Can you work these out from the model? Positions are in its coordinate system, mm. Face numbers are marked on the shaded views. A direction names the side the tool comes from. Round coordinates to 2 decimals unless told otherwise and drop trailing zeros. Loops run counter-clockwise (first coordinate to the right, second up) from the corner with the lowest first, then second, coordinate; pieces in that order, holes last.
(1) Thinking about a two-plate mould opening in Y: for the marked faces 4, 5 and 6, which applies, released by +Y, released by -Y, zero draft, split by the parting line, or undercut?
(2) I want a section at C-C on x = 0.4. Write out the boundary of the cut face in (y, z).
(3) I want a section at B-B on z = 0.3. Write out the boundary of the cut face in (x, y).
(4) If I drill on line 1 along Y through (x, z) = (0.2, -0.25); line 2 along Y through (x, z) = (-0.6, 1.8); line 3 along X through (y, z) = (-11, 0.8), over which ranges is the centre line in solid material (lowest first)?
(5) I want a section at D-D on y = 2. Write out the boundary of the cut face in (x, z), plus the area to 3 significant figures.
(6) I want a section at A-A on y = 9. Write out the boundary of the cut face in (x, z).
(7) Will these pins go through, and if not, where does the flat tip stop? pin 1 Ø1.7 at (x, y) = (0.2, -11) entering from +Z; pin 2 Ø0.8 at (x, z) = (-1.5, 1) entering from +Y; pin 3 Ø0.6 at (x, y) = (0, 8) entering from +Z.
(8) Which directions (+Z, -Z, +X, -X, +Y, -Y) give clear straight access to the entire face, cutting with the end or side of a thin tool? Please do the marked faces 1, 2 and 3.
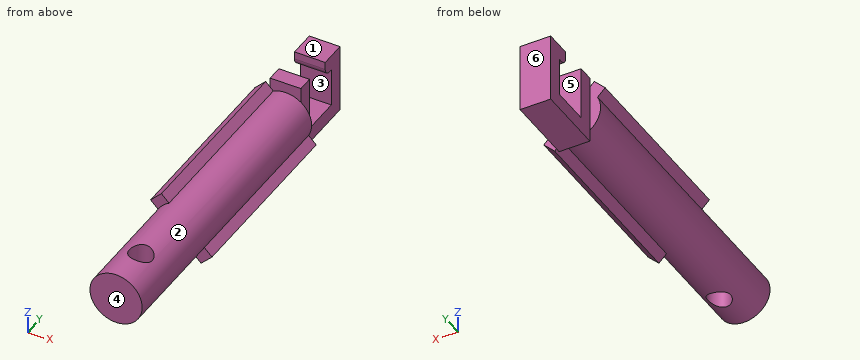
from build123d import *

# Parameters (mm, degrees)
SKETCH1_R             = 1.7
MAIN_SHAFT_DEPTH      = 6
GUIDES_DEPTH          = 12
SKETCH21_W            = 2
SKETCH21_H            = 4.5
HOOK_EXTRUDE_DEPTH    = 4.5
HOOK_CUT_DEPTH        = 3.997440667
HOOK_FILLET_R         = 0.5
SKETCH23_R            = 1.7
TOP_STOPPER_DEPTH     = 2
SKETCH24_R            = 1.7
BOTTOM_SHAFT_DEPTH    = 5.5
F_1_5MM_DOWEL_HOLE2_D = 1.5


with BuildPart() as part:
    # Sketch1 → main shaft (new body, symmetric)
    with BuildSketch(Plane(origin=(0, 0, 0), x_dir=(1, 0, 0), z_dir=(0, 1, 0))):
        Circle(SKETCH1_R)
    extrude(amount=MAIN_SHAFT_DEPTH, both=True)

    # Sketch2 → guides (add)
    with BuildSketch(Plane(origin=(0, 6, 0), x_dir=(1, 0, 0), z_dir=(0, 1, 0))):
        with BuildLine():
            Line((-0.795359139, -1.50246592), (-1.290333886, -1.997440667))
            Line((-1.290333886, -1.997440667), (-1.997440667, -1.290333886))
            Line((-1.997440667, -1.290333886), (-1.50246592, -0.795359139))
            ThreePointArc((-1.50246592, -0.795359139), (-1.202081528, -1.202081528), (-0.795359139, -1.50246592))
        make_face()
        with BuildLine():
            Line((1.290333886, 1.997440667), (0.795359139, 1.50246592))
            ThreePointArc((0.795359139, 1.50246592), (1.202081528, 1.202081528), (1.50246592, 0.795359139))
            Line((1.50246592, 0.795359139), (1.997440667, 1.290333886))
            Line((1.997440667, 1.290333886), (1.290333886, 1.997440667))
        make_face()
    extrude(amount=-GUIDES_DEPTH)

    # Sketch21 → hook extrude (add)
    with BuildSketch(Plane(origin=(0, 6, 0), x_dir=(1, 0, 0), z_dir=(0, 1, 0))):
        with Locations((0, -0.1)):
            Rectangle(SKETCH21_W, SKETCH21_H)
    extrude(amount=HOOK_EXTRUDE_DEPTH)

    # Sketch22 → hook cut (cut, through all)
    with BuildSketch(Plane(origin=(1, 0, 0), x_dir=(0, 0, -1), z_dir=(1, 0, 0))):
        Polygon((-2.35, 7), (1.15, 7), (1.15, 9.5), (-1.35, 9.5), (-1.35, 8.8), (-2.35, 8.8), align=None)
    extrude(amount=-HOOK_CUT_DEPTH, mode=Mode.SUBTRACT)

    # hook fillet
    hook_fillet_edges = [part.edges().sort_by_distance(p)[0] for p in [
        (0, 8.8, 1.35),
    ]]
    fillet(hook_fillet_edges, radius=HOOK_FILLET_R)

    # Sketch23 → top stopper (add)
    with BuildSketch(Plane.XZ.offset(6)):
        Circle(SKETCH23_R)
    extrude(amount=TOP_STOPPER_DEPTH)

    # Sketch24 → bottom shaft (add)
    with BuildSketch(Plane.XZ.offset(8)):
        Circle(SKETCH24_R)
    extrude(amount=BOTTOM_SHAFT_DEPTH)

    # Ø1.5mm Dowel Hole2 (through all)
    with Locations(Plane.XY.offset(2.35)):
        with Locations((0.2, -11)):
            Hole(F_1_5MM_DOWEL_HOLE2_D / 2)


solid = part.part
Filled sheet:
1. face 4: released by -Y
1. face 5: undercut
1. face 6: released by +Y
2. outline: (-13.5, -1.65) - (-11.72, -1.65) - (-11.72, 1.65) - (-13.5, 1.65) - close; (-10.28, -1.65) - (6, -1.65) - (6, -2.15) - (10.5, -2.15) - (10.5, 2.35) - (8.8, 2.35) - (8.8, 1.85) arc R0.5 ccw to (9.3, 1.35) - (9.5, 1.35) - (9.5, -1.15) - (7, -1.15) - (7, 2.35) - (6, 2.35) - (6, 1.65) - (-10.28, 1.65) - close
3. outline: (-1.67, -13.5) - (1.67, -13.5) - (1.67, 6) - (1, 6) - (1, 7) - (-1, 7) - (-1, 6) - (-1.67, 6) - close; (-1, 9.5) - (1, 9.5) - (1, 10.5) - (-1, 10.5) - close; hole circle Ø1.5 at (0.2, -11)
4. line 1: y = -13.5 to -11.75, -10.25 to 7, 9.5 to 10.5
4. line 2: y = 6 to 7, 8.8 to 10.5
4. line 3: x = -1.5 to -0.55, 0.95 to 1.5
5. outline: (-2, 1.29) - (-1.5, 0.8) arc R1.7 ccw to (0.8, -1.5) - (1.29, -2) - (2, -1.29) - (1.5, -0.8) arc R1.7 ccw to (-0.8, 1.5) - (-1.29, 2) - close
5. area: 10.4 mm2
6. outline: (-1, -2.15) - (1, -2.15) - (1, -1.15) - (-1, -1.15) - close; (-1, 1.45) - (1, 1.45) - (1, 2.35) - (-1, 2.35) - close
7. pin 1: stops at z = 1.7
7. pin 2: stops at y = 6
7. pin 3: stops at z = -1.15
8. face 1: +Z, +X, -X, +Y, -Y
8. face 2: -Y
8. face 3: +X, -X
